Check sheet for the modelled part. Datum: model origin and axes. Units: mm. A direction names the side the tool comes from. Give positions to 0.01 mm unless a question says otherwise; leave off trailing zeros. Order: outer loops, then holes, each group sorted by start corner. A loop starts at its lowest first (then second) coordinate and runs counter-clockwise, first axis right, second up. Notation, with made-up numbers: M 16,21 L 44,21 A10 cw 44,37 Z; hole C 1,38.25 d10. An arc over 180 degrees is marked long. One line per question, with ' | ' between items. Start each with the question number.
Autodesk Inventor part; units mm, degrees
ref_plane "YZ Plane" through (0, 0, 0) normal (1, 0, 0) x (0, 1, 0)
ref_plane "XZ Plane" through (0, 0, 0) normal (0, 1, 0) x (-1, 0, 0)
ref_plane "XY Plane" through (0, 0, 0) normal (0, 0, 1) x (1, 0, 0)
ref_plane "Work Plane1" through (0, 0, 8) normal (0, 0, 1) x (1, 0, 0)
sketch "Sketch1" plane through (0, 0, 0) normal (0, 0, 1) x (1, 0, 0)
  circle A0 centre (0, 0) radius 2.6023
  line L0 (-0.1767, 8.453) -> (0.1689, 8.453)
  line L1 (0.1689, 8.453) -> (0.9579, 5.5085) construction
  arc A1 (-0.1767, 8.453) -> (-0.9656, 5.5084) centre (2.8217, 6.0717) ccw
  line L2 (-5.1115, 6.7348) -> (-4.8319, 6.9379)
  arc A2 (-2.4629, 5.0195) -> (-4.8319, 6.9379) centre (-5.8579, 3.249) ccw
  line L3 (-4.8319, 6.9379) -> (-2.4629, 5.0195) construction
  arc A3 (-5.1115, 6.7348) -> (-4.0189, 3.8888) centre (-1.286, 6.5706) ccw
  line L4 (-8.0939, 2.4441) -> (-7.9871, 2.7727)
  arc A4 (-4.9429, 2.6132) -> (-7.9871, 2.7727) centre (-6.6488, -0.8147) ccw
  line L5 (-7.9871, 2.7727) -> (-4.9429, 2.6132) construction
  arc A5 (-8.0939, 2.4441) -> (-5.5371, 0.7838) centre (-4.9025, 4.5598) ccw
  line L6 (-7.9847, -2.7801) -> (-8.0915, -2.4515)
  arc A6 (-5.5349, -0.7913) -> (-8.0915, -2.4515) centre (-4.9001, -4.5672) ccw
  line L7 (-8.0915, -2.4515) -> (-5.5349, -0.7913) construction
  arc A7 (-7.9847, -2.7801) -> (-4.9404, -2.6205) centre (-6.6464, 0.8073) ccw
  line L8 (-4.8256, -6.9425) -> (-5.1052, -6.7393)
  arc A8 (-4.0128, -3.8935) -> (-5.1052, -6.7393) centre (-1.2798, -6.5752) ccw
  line L9 (-5.1052, -6.7393) -> (-4.0128, -3.8935) construction
  line L10 (0.1767, -8.453) -> (-0.1689, -8.453)
  arc A9 (-0.9579, -5.5085) -> (-0.1689, -8.453) centre (2.8295, -6.0717) ccw
  line L11 (-0.1689, -8.453) -> (-0.9579, -5.5085) construction
  arc A10 (0.1767, -8.453) -> (0.9656, -5.5084) centre (-2.8217, -6.0717) ccw
  line L12 (5.1115, -6.7348) -> (4.8319, -6.9379)
  arc A11 (2.4629, -5.0195) -> (4.8319, -6.9379) centre (5.8579, -3.249) ccw
  line L13 (4.8319, -6.9379) -> (2.4629, -5.0195) construction
  arc A12 (5.1115, -6.7348) -> (4.0189, -3.8888) centre (1.286, -6.5706) ccw
  line L14 (8.0939, -2.4441) -> (7.9871, -2.7727)
  arc A13 (3.3182, -1.074) -> (8.2332, -2.671) centre (6.6488, 0.8147) ccw
  line L15 (7.9871, -2.7727) -> (4.9429, -2.6132) construction
  line L16 (7.9847, 2.7801) -> (8.0915, 2.4515)
  arc A14 (5.5349, 0.7913) -> (8.0915, 2.4515) centre (4.9001, 4.5672) ccw
  line L17 (8.0915, 2.4515) -> (4.0908, -0.1465) construction
  arc A15 (7.9847, 2.7801) -> (4.9404, 2.6205) centre (6.6464, -0.8073) ccw
  line L18 (4.8256, 6.9425) -> (5.1052, 6.7393)
  arc A16 (4.0128, 3.8935) -> (5.1052, 6.7393) centre (1.2798, 6.5752) ccw
  line L19 (5.1052, 6.7393) -> (4.0128, 3.8935) construction
  arc A17 (-5.5371, 0.7838) -> (-5.536, -0.7919) centre (0, 0) ccw
  arc A18 (-4.0189, 3.8888) -> (-4.9442, 2.6133) centre (0, 0) ccw
  arc A19 (2.4565, 5.0239) -> (0.9575, 5.5098) centre (0, 0) ccw
  arc A20 (4.9404, 2.6205) -> (4.0132, 3.8947) centre (0, 0) ccw
  arc A21 (4.9442, -2.6133) -> (5.536, 0.7919) centre (0, 0) ccw
  arc A22 (2.4639, -5.0203) -> (4.9442, -2.6133) centre (0, 0) ccw
  arc A23 (0.9656, -5.5084) -> (2.4639, -5.0203) centre (0, 0) ccw
  arc A24 (-4.9404, -2.6205) -> (-4.0132, -3.8947) centre (0, 0) ccw
  arc A25 (-2.4565, -5.0239) -> (-0.9575, -5.5098) centre (0, 0) ccw
  arc A26 (0.9579, 5.5085) -> (0.1689, 8.453) centre (-2.8295, 6.0717) ccw
  arc A27 (-2.1474, 2.3039) -> (-1.5764, 2.4536) centre (-2.8295, 6.0717) ccw
  arc A28 (-3.1006, 2.2523) -> (-3.0363, 2.2483) centre (-2.8295, 6.0717) ccw
  arc A29 (4.8256, 6.9425) -> (2.4565, 5.0239) centre (5.8516, 3.2535) ccw
  circle A30 centre (4.9025, -4.5598) radius 3.829
  arc A31 (1.7403, -2.4009) -> (1.7114, -2.4439) centre (4.9025, -4.5598) ccw
  arc A32 (1.1846, -3.6447) -> (1.1248, -3.9359) centre (4.9025, -4.5598) ccw
  arc A33 (-4.8256, -6.9425) -> (-2.4565, -5.0239) centre (-5.8516, -3.2535) ccw
  arc A34 (-2.1424, -2.3034) -> (-2.3452, -1.7153) centre (-5.8516, -3.2535) ccw
  arc A35 (-0.9656, 5.5084) -> (-2.4639, 5.0203) centre (0, 0) ccw
  arc A36 (-4.0189, 3.8888) -> (-4.9442, 2.6133) centre (0, 0) ccw
  point P0 (-0.7682, 6.1639)
  point P1 (0.7605, 6.1646)
  point P2 (-4.2445, 4.5351)
  point P3 (-3.0082, 5.4342)
  point P4 (-6.0996, 1.1741)
  point P5 (-5.6279, 2.6282)
  point P6 (-5.6248, -2.6354)
  point P7 (-6.0979, -1.1817)
  point P8 (-3.0015, -5.4382)
  point P9 (-4.2387, -4.5403)
  point P10 (0.7682, -6.1639)
  point P11 (-0.7605, -6.1646)
  point P12 (4.2445, -4.5351)
  point P13 (3.0082, -5.4342)
  point P14 (6.0996, -1.1741)
  point P15 (5.6279, -2.6282)
  point P16 (5.6248, 2.6354)
  point P17 (6.0979, 1.1817)
  point P18 (3.0015, 5.4382)
  point P19 (4.2387, 4.5403)
sketch "Sketch2" plane through (0, 0, 8) normal (0, 0, 1) x (1, 0, 0)
  circle A0 centre (0, 0) radius 2.6023
  arc A1 (-5.2272, 2.3957) -> (-5.6389, 1.125) centre (0, 0) ccw
  circle A2 centre (0, 0) radius 8.8963
  dimension "d8" = 17.7926
extrude "Extrusion2" add sketch "Sketch2" along normal blind 8.85
ref_plane "Work Plane2" through (0, 0, 16.85) normal (0, 0, 1) x (1, 0, 0)
sketch "Sketch3" plane through (0, 0, 16.85) normal (0, 0, 1) x (1, 0, 0)
  circle A0 centre (0, 0) radius 2.6023
  circle A1 centre (0, 0) radius 8.8963
  line L0 (0, 6.8373) -> (3.0745, 6.8373)
  line L1 (3.0745, 6.8373) -> (3.0745, 4.6023)
  line L2 (3.0745, 4.6023) -> (0, 4.6023)
  line L3 (0, 6.8373) -> (-3.0745, 6.8373)
  line L4 (-3.0745, 6.8373) -> (-3.0745, 4.6023)
  line L5 (-3.0745, 4.6023) -> (0, 4.6023)
  line L6 (0, -4.8344) -> (3.0745, -4.8344)
  line L7 (3.0745, -4.8344) -> (3.0745, -7.0696)
  line L8 (3.0745, -7.0696) -> (0, -7.0696)
  line L9 (0, -4.8344) -> (-3.0745, -4.8344)
  line L10 (-3.0745, -4.8344) -> (-3.0745, -7.0696)
  line L11 (-3.0745, -7.0696) -> (0, -7.0696)
  line L12 (0, -9.0696) -> (0, -7.0696)
  line L13 (0, 2.6023) -> (0, 3.7788)
  line L14 (0, 3.7788) -> (0, 4.6023)
  dimension "d10" = 2.235
  dimension "d11" = 2
  dimension "d31" = 2.2352
  dimension "d32" = 6.149
  dimension "d33" = 6.149
extrude "Extrusion3" cut sketch "Sketch3" against normal blind 8 contours L5 L4 L3 L0 L1 L2
ref_plane "Work Plane3" through (-2.75, 6.6023, 16.85) normal (0, -1, 0) x (1, 0, 0)
sketch "Sketch4" plane through (-2.75, 6.6023, 16.85) normal (0, -1, 0) x (1, 0, 0)
  line L0 (5.5, 0) -> (5.5, -8)
  line L1 (2.75, 0.553) -> (2.75, -3.197)
  circle A0 centre (2.75, -2.8775) radius 1.75
  point P0 (2.75, -16.85)
  dimension "d14" = 3.75
  dimension "d15" = 3.5
extrude "Extrusion4" cut sketch "Sketch4" along normal mid plane 9
sketch "Sketch5" plane through (0, 0, 8) normal (0, 0, -1) x (-1, 0, 0)
  circle A0 centre (0, 0) radius 2.6023
  circle A1 centre (0, 0) radius 8.8963
  line L0 (-0.1767, 8.453) -> (0.169, 8.453)
  line L1 (0.1689, 8.453) -> (0.9579, 5.5085) construction
  arc A2 (0.9579, 5.5085) -> (0.1689, 8.453) centre (-2.8295, 6.0717) ccw
  circle A3 centre (0, 0) radius 2.6023
  arc A4 (-0.1767, 8.453) -> (-0.9656, 5.5085) centre (2.8217, 6.0717) ccw
  arc A5 (0.9575, 5.5099) -> (0.169, 8.453) centre (-2.8254, 6.0736) ccw
  line L2 (0.1689, 8.453) -> (-0.1767, 8.453)
  arc A6 (-0.1767, 8.453) -> (-0.9656, 5.5085) centre (2.8217, 6.0717) ccw
  line L3 (-5.1115, 6.7348) -> (-4.8318, 6.9379)
  line L4 (-4.8319, 6.9379) -> (-2.4629, 5.0195) construction
  arc A7 (-2.4629, 5.0195) -> (-4.8319, 6.9379) centre (-5.8579, 3.249) ccw
  arc A8 (-5.1115, 6.7348) -> (-4.019, 3.8889) centre (-1.286, 6.5706) ccw
  arc A9 (-2.464, 5.0204) -> (-4.8318, 6.9379) centre (-5.8558, 3.2529) ccw
  line L5 (-4.8319, 6.9379) -> (-5.1115, 6.7348)
  arc A10 (-5.1115, 6.7348) -> (-4.019, 3.8889) centre (-1.286, 6.5706) ccw
  line L6 (-8.0939, 2.4441) -> (-7.987, 2.7728)
  line L7 (-7.9871, 2.7727) -> (-4.9429, 2.6132) construction
  arc A11 (-4.9429, 2.6132) -> (-7.9871, 2.7727) centre (-6.6488, -0.8147) ccw
  arc A12 (-8.0939, 2.4441) -> (-5.5373, 0.7839) centre (-4.9025, 4.5598) ccw
  arc A13 (-4.9444, 2.6133) -> (-7.987, 2.7728) centre (-6.6494, -0.8103) ccw
  line L8 (-7.9871, 2.7727) -> (-8.0939, 2.4441)
  arc A14 (-8.0939, 2.4441) -> (-5.5373, 0.7839) centre (-4.9025, 4.5598) ccw
  line L9 (-7.9847, -2.7801) -> (-8.0915, -2.4514)
  line L10 (-8.0915, -2.4515) -> (-5.5349, -0.7913) construction
  arc A15 (-5.5349, -0.7913) -> (-8.0915, -2.4515) centre (-4.9001, -4.5672) ccw
  arc A16 (-7.9847, -2.7801) -> (-4.9405, -2.6206) centre (-6.6464, 0.8073) ccw
  arc A17 (-5.5361, -0.792) -> (-8.0915, -2.4514) centre (-4.9032, -4.564) ccw
  line L11 (-8.0915, -2.4515) -> (-7.9847, -2.7801)
  arc A18 (-7.9847, -2.7801) -> (-4.9405, -2.6206) centre (-6.6464, 0.8073) ccw
  line L12 (-4.8256, -6.9425) -> (-5.1053, -6.7393)
  line L13 (-5.1052, -6.7393) -> (-4.0128, -3.8935) construction
  arc A19 (-4.0128, -3.8935) -> (-5.1052, -6.7393) centre (-1.2798, -6.5752) ccw
  arc A20 (-4.8256, -6.9425) -> (-2.4566, -5.0241) centre (-5.8516, -3.2535) ccw
  arc A21 (-4.0133, -3.8948) -> (-5.1053, -6.7393) centre (-1.2842, -6.5744) ccw
  line L14 (-5.1052, -6.7393) -> (-4.8256, -6.9425)
  arc A22 (-4.8256, -6.9425) -> (-2.4566, -5.0241) centre (-5.8516, -3.2535) ccw
  line L15 (0.1767, -8.453) -> (-0.169, -8.453)
  line L16 (-0.1689, -8.453) -> (-0.9579, -5.5085) construction
  arc A23 (-0.9579, -5.5085) -> (-0.1689, -8.453) centre (2.8295, -6.0717) ccw
  arc A24 (0.1767, -8.453) -> (0.9656, -5.5085) centre (-2.8217, -6.0717) ccw
  arc A25 (-0.9575, -5.5099) -> (-0.169, -8.453) centre (2.8254, -6.0736) ccw
  line L17 (-0.1689, -8.453) -> (0.1767, -8.453)
  arc A26 (0.1767, -8.453) -> (0.9656, -5.5085) centre (-2.8217, -6.0717) ccw
  line L18 (5.1115, -6.7348) -> (4.8318, -6.9379)
  line L19 (4.8319, -6.9379) -> (2.4629, -5.0195) construction
  arc A27 (2.4629, -5.0195) -> (4.8319, -6.9379) centre (5.8579, -3.249) ccw
  arc A28 (5.1115, -6.7348) -> (4.019, -3.8889) centre (1.286, -6.5706) ccw
  arc A29 (2.464, -5.0204) -> (4.8318, -6.9379) centre (5.8558, -3.2529) ccw
  line L20 (4.8319, -6.9379) -> (5.1115, -6.7348)
  arc A30 (5.1115, -6.7348) -> (4.019, -3.8889) centre (1.286, -6.5706) ccw
  line L21 (8.0939, -2.4441) -> (7.987, -2.7728)
  line L22 (7.9871, -2.7727) -> (4.9429, -2.6132) construction
  arc A31 (4.9429, -2.6132) -> (7.9871, -2.7727) centre (6.6488, 0.8147) ccw
  arc A32 (8.0939, -2.4441) -> (5.5373, -0.7839) centre (4.9025, -4.5598) ccw
  arc A33 (4.9444, -2.6133) -> (7.987, -2.7728) centre (6.6494, 0.8103) ccw
  line L23 (7.9871, -2.7727) -> (8.0939, -2.4441)
  arc A34 (8.0939, -2.4441) -> (5.5373, -0.7839) centre (4.9025, -4.5598) ccw
  line L24 (7.9847, 2.7801) -> (8.0915, 2.4514)
  line L25 (8.0915, 2.4515) -> (5.5349, 0.7913) construction
  arc A35 (5.5349, 0.7913) -> (8.0915, 2.4515) centre (4.9001, 4.5672) ccw
  arc A36 (7.9847, 2.7801) -> (4.9405, 2.6206) centre (6.6464, -0.8073) ccw
  arc A37 (5.5361, 0.792) -> (8.0915, 2.4514) centre (4.9032, 4.564) ccw
  line L26 (8.0915, 2.4515) -> (7.9847, 2.7801)
  arc A38 (7.9847, 2.7801) -> (4.9405, 2.6206) centre (6.6464, -0.8073) ccw
  line L27 (4.8256, 6.9425) -> (5.1053, 6.7393)
  line L28 (5.1052, 6.7393) -> (4.0128, 3.8935) construction
  arc A39 (4.0128, 3.8935) -> (5.1052, 6.7393) centre (1.2798, 6.5752) ccw
  arc A40 (4.8256, 6.9425) -> (2.4566, 5.0241) centre (5.8516, 3.2535) ccw
  arc A41 (4.0133, 3.8948) -> (5.1053, 6.7393) centre (1.2842, 6.5744) ccw
  line L29 (5.1052, 6.7393) -> (4.8256, 6.9425)
  arc A42 (4.8256, 6.9425) -> (2.4566, 5.0241) centre (5.8516, 3.2535) ccw
  arc A43 (2.4566, 5.0241) -> (0.9575, 5.5099) centre (0, 0) ccw
  arc A44 (4.9405, 2.6206) -> (4.0133, 3.8948) centre (0, 0) ccw
  arc A45 (5.5373, -0.7839) -> (5.5361, 0.792) centre (0, 0) ccw
  arc A46 (4.019, -3.8889) -> (4.9444, -2.6133) centre (0, 0) ccw
  arc A47 (0.9656, -5.5085) -> (2.464, -5.0204) centre (0, 0) ccw
  arc A48 (-2.4566, -5.0241) -> (-0.9575, -5.5099) centre (0, 0) ccw
  arc A49 (-4.9405, -2.6206) -> (-4.0133, -3.8948) centre (0, 0) ccw
  arc A50 (-5.5373, 0.7839) -> (-5.5361, -0.792) centre (0, 0) ccw
  arc A51 (-0.9656, 5.5085) -> (-2.464, 5.0204) centre (0, 0) ccw
  arc A52 (-4.019, 3.8889) -> (-4.9444, 2.6133) centre (0, 0) ccw
  point P0 (-0.7682, 6.1639)
  point P1 (0.7605, 6.1646)
  point P2 (-1.286, 6.5706)
  point P3 (1.2798, 6.5752)
  point P4 (0.9575, 5.5098)
  point P5 (-4.9025, 4.5598)
  point P6 (-4.2445, 4.5351)
  point P7 (-2.4639, 5.0203)
  point P8 (-3.0082, 5.4342)
  point P9 (-2.8295, 6.0717)
  point P10 (-6.6464, 0.8073)
  point P11 (-6.0996, 1.1741)
  point P12 (-4.9442, 2.6133)
  point P13 (-5.6279, 2.6282)
  point P14 (-5.8579, 3.249)
  point P15 (-5.8516, -3.2535)
  point P16 (-5.6248, -2.6354)
  point P17 (-5.536, -0.7919)
  point P18 (-6.0979, -1.1817)
  point P19 (-6.6488, -0.8147)
  point P20 (-2.8217, -6.0717)
  point P21 (-3.0015, -5.4382)
  point P22 (-4.0132, -3.8947)
  point P23 (-4.2387, -4.5403)
  point P24 (-4.9001, -4.5672)
  point P25 (1.286, -6.5706)
  point P26 (0.7682, -6.1639)
  point P27 (-0.9575, -5.5098)
  point P28 (-0.7605, -6.1646)
  point P29 (-1.2798, -6.5752)
  point P30 (4.9025, -4.5598)
  point P31 (4.2445, -4.5351)
  point P32 (2.4639, -5.0203)
  point P33 (3.0082, -5.4342)
  point P34 (2.8295, -6.0717)
  point P35 (6.6464, -0.8073)
  point P36 (6.0996, -1.1741)
  point P37 (4.9442, -2.6133)
  point P38 (5.6279, -2.6282)
  point P39 (5.8579, -3.249)
  point P40 (5.8516, 3.2535)
  point P41 (5.6248, 2.6354)
  point P42 (5.536, 0.7919)
  point P43 (6.0979, 1.1817)
  point P44 (6.6488, 0.8147)
  point P45 (2.8217, 6.0717)
  point P46 (3.0015, 5.4382)
  point P47 (4.0132, 3.8947)
  point P48 (4.2387, 4.5403)
  point P49 (4.9001, 4.5672)
  dimension "d27" = 360
extrude "Extrusion5" add sketch "Sketch5" along normal blind 10 contours L0 A2 A43 A40 L27 A39 A44 A36 L24 A35 A45 A32 L21 A31 A46 A28 L18 A27 A47 A24 L15 A23 A48 A20 L12 A19 A49 A16 L9 A15 A50 A12 L6 A11 A52 A8 L3 A7 A51 A4
properties part number "sj-small-gear"
Item 1: Section check B-B, the plane z = 11.5. Record the cut outline in (x, y).
Item 2: Draft check along X on faces 4 (the face through (-6.97, -1.337, 3.07)), 5 (the face through (-1.742, -5.314, 3.07)), 6 (the face through (6.97, 1.337, 3.07)). Enter one of: released by +X, released by -X, zero draft, split by the parting line, or undercut.
Item 3: Section check C-C, the plane x = -7. Record the cut outline in (y, z).
Item 4: Go/stop test with flat-tipped pins: P1, Ø1.5, axis at x = -3.5, z = 4.5, coming from the +Y side; P2, Ø4, axis at y = 6.5, z = 5.5, coming from the -X side; P3, Ø1.5, axis at x = -2, z = 11, coming from the -Y side. Record where each tip stops, or that it passes through.
Item 5: Set-up check for faces 1 (the face through (3.47, 6.24, 3.07)), 2 (the face through (5.592, -0.015, 3.07)), 3 (the face through (-4.53, -3.28, 3.07)): record each of +Z, -Z, +X, -X, +Y, -Y from which the full face is reachable in a straight line by a thin tool's end or side.
Item 6: Scan lines: probe 1 along Y at (x, z) = (0, 2.75); probe 2 along Z at (x, y) = (0, 3.6); probe 3 along Y at (x, z) = (2, 12.25). Record each from-to range of solid material in increasing order. Write a range as [from, to].
Item 7: Section check A-A, the plane y = 0. Record the cut outline in (x, z), then the cut area to 3 significant figures.
Item 8: Section check D-D, the plane x = 4.5. Record the cut outline in (y, z).
Reported:
1) outline: C 0,0 d17.79; hole M -3.07,4.6 L 3.07,4.6 L 3.07,6.84 L -3.07,6.84 Z; hole C 0,0 d5.2
2) face 4: released by -X | face 5: undercut | face 6: released by +X
3) outline: M -5.49,8 L -3,8 L -3,-2 L -1.36,-2 L -1.36,8 L 1.37,8 L 1.37,-2 L 3.01,-2 L 3.01,8 L 5.49,8 L 5.49,16.85 L -5.49,16.85 Z
4) P1: stops at y = 6.73 | P2: stops at x = -5.11 | P3: stops at y = -8.81
5) face 1: -Z, +Y | face 2: -Z, +X | face 3: -Z
6) probe 1: y = [-8.45, -2.6], [2.6, 8.45] | probe 2: z = [-2, 12.22], [15.72, 16.85] | probe 3: y = [-8.67, -1.66], [1.66, 4.6], [6.84, 8.67]
7) outline: M -8.9,8 L -5.59,8 L -5.59,-2 L -2.6,-2 L -2.6,16.85 L -8.9,16.85 Z; M 2.6,-2 L 5.59,-2 L 5.59,8 L 8.9,8 L 8.9,16.85 L 2.6,16.85 Z | area: 171 mm^2
8) outline: M -7.67,8 L -6.84,8 L -6.84,-2 L -4.5,-2 L -4.5,8 L -3.32,8 L -3.32,-2 L 3.32,-2 L 3.32,8 L 4.49,8 L 4.49,-2 L 6.83,-2 L 6.83,8 L 7.67,8 L 7.67,16.85 L -7.67,16.85 Z
